Check sheet for the drawn part. Datum: minimum x, y, z corner. Units: mm. A direction names the side the tool comes from. Round coordinates to 2 decimals unless told otherwise and drop trailing zeros. Order: outer loops, then holes, each group sorted by start corner. A loop starts at its lowest first (then second) coordinate and runs counter-clockwise, first axis right, second up. Notation, with made-up numbers: M 39,54 L 87,54 A15 ccw 87,61 Z; hole C -5,70.5 d5. An arc over 180 degrees is marked long. Answer as a JSON object with one key per item and string values. Group by question number.
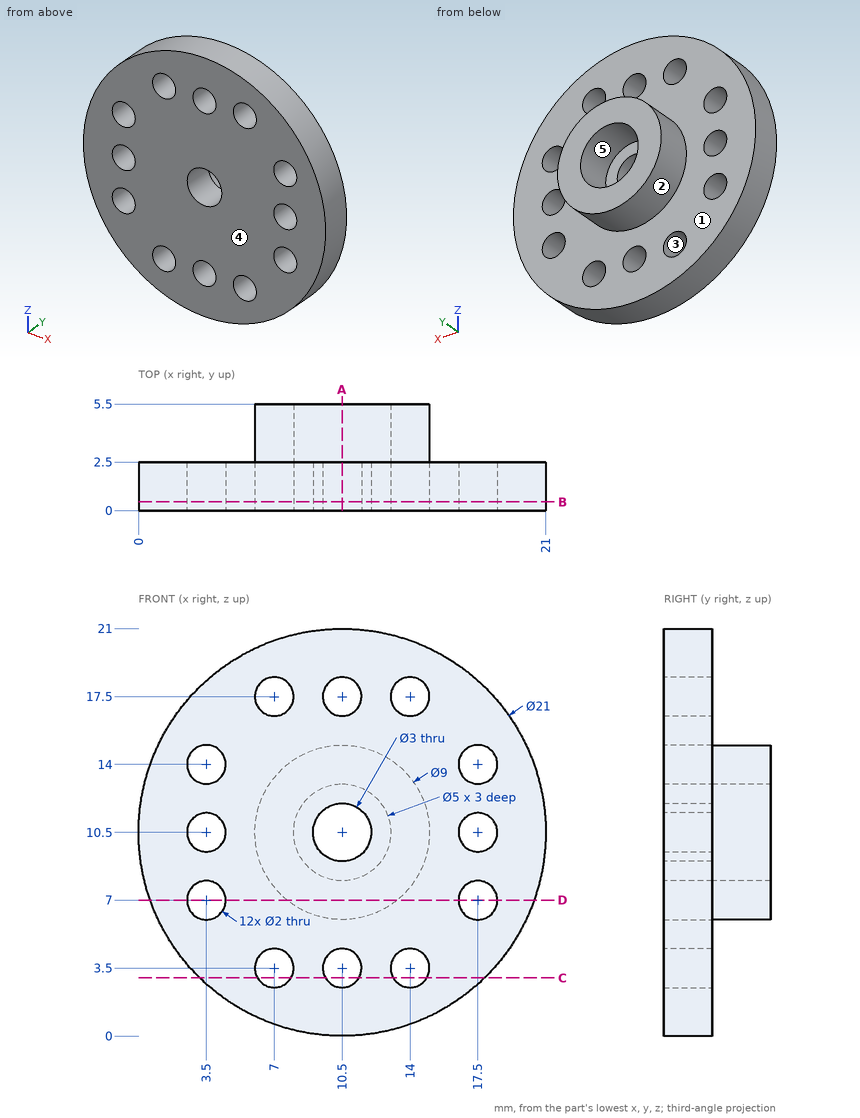
1) Go/stop test with flat-tipped pins: P1, Ø2.5, axis at x = 11, z = 10.5, coming from the +Y side; P2, Ø1, axis at y = 3.5, z = 18, coming from the +X side; P3, Ø2, axis at y = 4.5, z = 9.5, coming from the +X side. Record where each tip stops, or that it passes through.
2) Thickness scan on line 1 along X through (y, z) = (1.55, 10.5); line 2 along X through (y, z) = (1.6, 3.5); line 3 along Z through (x, y) = (4, 0.6). Record the ranges inside material, lowest first. Write a range as [from, to].
3) Sectioned sample at A-A (x = 10.5). Record the boundary of the cut face in (y, z).
4) Set-up check for the marked faces 4 and 5: record each of +Z, -Z, +X, -X, +Y, -Y from which the full face is reachable in a straight line by a thin tool's end or side.
5) Sectioned sample at B-B (y = 0.45). Count the separate pieces of the cut face and the enclosed holes in it, then the cut area to 3 significant figures.
6) Release check for a two-part mould opening along Z. For the marked faces 1, 2 and 3 record: +Z half, -Z half, draft (parallel to the pull), parting line (faces both ways), or undercut.
7) Sectioned sample at D-D (z = 7). Record the boundary of the cut face in (x, y), then the cut area to 3 significant figures.
8) Sectioned sample at C-C (z = 3). Record the boundary of the cut face in (x, y).
Final values:
{
 "1": {"P1": "stops at y = 2.5", "P2": "passes through", "P3": "stops at x = 15"},
 "2": {"line 1": "x = [0, 2.5], [4.5, 9], [12, 16.5], [18.5, 21]", "line 2": "x = [2.67, 6], [8, 9.5], [11.5, 13], [15, 18.33]", "line 3": "z = [2.25, 6.13], [7.87, 9.63], [11.37, 13.13], [14.87, 18.75]"},
 "3": {"outline": "M 0,0 L 2.5,0 L 2.5,2.5 L 0,2.5 Z; M 0,4.5 L 2.5,4.5 L 2.5,6 L 5.5,6 L 5.5,8 L 2.5,8 L 2.5,9 L 0,9 Z; M 0,12 L 2.5,12 L 2.5,13 L 5.5,13 L 5.5,15 L 2.5,15 L 2.5,16.5 L 0,16.5 Z; M 0,18.5 L 2.5,18.5 L 2.5,21 L 0,21 Z"},
 "4": {"face 4": "+Z, -Z, +X, -X, -Y", "face 5": "+Y"},
 "5": {"separate pieces": "1", "enclosed holes": "13", "area": "302 mm^2"},
 "6": {"face 1": "draft", "face 2": "parting line", "face 3": "undercut"},
 "7": {"outline": "M 0.6,0 L 2.5,0 L 2.5,2.5 L 0.6,2.5 Z; M 4.5,0 L 16.5,0 L 16.5,2.5 L 13.33,2.5 L 13.33,5.5 L 7.67,5.5 L 7.67,2.5 L 4.5,2.5 Z; M 18.5,0 L 20.4,0 L 20.4,2.5 L 18.5,2.5 Z", "area": "56.5 mm^2"},
 "8": {"outline": "M 3.15,0 L 6.13,0 L 6.13,2.5 L 3.15,2.5 Z; M 7.87,0 L 9.63,0 L 9.63,2.5 L 7.87,2.5 Z; M 11.37,0 L 13.13,0 L 13.13,2.5 L 11.37,2.5 Z; M 14.87,0 L 17.85,0 L 17.85,2.5 L 14.87,2.5 Z"}
}
